Part model, mm, in its own coordinate system. Face numbers are marked on the shaded views. A direction names the side the tool comes from. Round coordinates to 2 decimals unless told otherwise and drop trailing zeros. Order: outer loops, then holes, each group sorted by start corner. A loop starts at its lowest first (then second) coordinate and runs counter-clockwise, first axis right, second up. Notation, with made-up numbers: (-28, -10.5) - (3, -10.5) arc R28 cw to (3, 21.5) - close; hole circle Ø1 at (0, 50.5). An arc over 180 degrees is marked (long way). Answer as a JSON object with one key per item and string values.
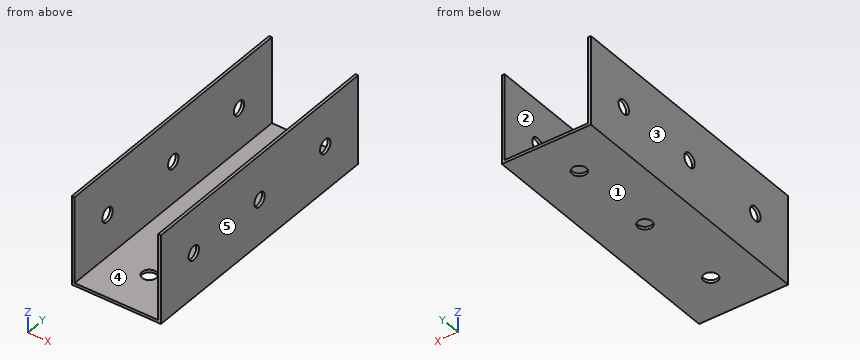
```python
from build123d import *

# Parameters (mm, degrees)
F1_DEPTH = 96
F2_R     = 2.54
F3_DEPTH = 50.8
F4_R     = 2.54
F5_DEPTH = 50.8
F6_R     = 2.54
F7_DEPTH = 25.4


with BuildPart() as f1:
    # F0 (on Front) → F1 (new body)
    with BuildSketch(Plane.XZ):
        Polygon((-15, 15.75), (-16, 15.75), (-16, -16.25), (16, -16.25), (16, 15.75), (15, 15.75), (15, -15.25), (-15, -15.25), align=None)
    extrude(amount=F1_DEPTH)

    # F2 (on face) → F3 (cut)
    with BuildSketch(Plane(origin=(-16, 0, 0), x_dir=(0, -1, 0), z_dir=(-1, 0, 0))):
        with Locations((16, -0.25)):
            Circle(F2_R)
    extrude(amount=-F3_DEPTH, mode=Mode.SUBTRACT)

    # F4 (on face) → F5 (cut)
    with BuildSketch(Plane(origin=(-16, 0, 0), x_dir=(0, -1, 0), z_dir=(-1, 0, 0))):
        with Locations((48, -0.25)):
            Circle(F4_R)
        with Locations((80, -0.25)):
            Circle(F4_R)
    extrude(amount=-F5_DEPTH, mode=Mode.SUBTRACT)

    # F6 (on face) → F7 (cut)
    with BuildSketch(Plane(origin=(0, 0, -16.25), x_dir=(1, 0, 0), z_dir=(0, 0, -1))):
        with Locations((0, 80)):
            Circle(F6_R)
        with Locations((0, 48)):
            Circle(F6_R)
        with Locations((0, 16)):
            Circle(F6_R)
    extrude(amount=-F7_DEPTH, mode=Mode.SUBTRACT)


solid = f1.part
```
Item 1: Cut at C-C (y = -48). Write the cut outline in (x, z), plus the area to 3 significant figures.
Taken from the geometry:
{"outline": "(-16, -16.25) - (-2.54, -16.25) - (-2.54, -15.25) - (-15, -15.25) - (-15, -2.79) - (-16, -2.79) - close; (-16, 2.29) - (-15, 2.29) - (-15, 15.75) - (-16, 15.75) - close; (2.54, -16.25) - (16, -16.25) - (16, -2.79) - (15, -2.79) - (15, -15.25) - (2.54, -15.25) - close; (15, 2.29) - (16, 2.29) - (16, 15.75) - (15, 15.75) - close", "area": "78.8 mm2"}
Item 2: Drop flat-ended pins along their axis: P1, Ø10, axis at y = -46, z = -1, coming from the -X side; P2, Ø6, axis at x = 0, y = -16, coming from the +Z side; P3, Ø3, axis at x = -12, z = 5, coming from the -Y side. Give the stop position or say it passes through.
Taken from the geometry:
{"P1": "x = -16", "P2": "z = -15.25", "P3": "through"}
Item 3: Two-plate mould, pull along X, no slides. Class the marked faces 1, 2 and 3: pulls with the +X half, pulls with the -X half, needs draft (parallel to the pull), parting line crosses it, or undercut.
Taken from the geometry:
{"face 1": "needs draft", "face 2": "undercut", "face 3": "pulls with the -X half"}
Item 4: Probe L1, parallel to Y at x = 0, z = -15.8; L2, parallel to X at y = -16, z = -16; L3, parallel to X at y = -19, z = -13. List the from-to ranges inside material, lowest first. Write a range as from..to.
Taken from the geometry:
{"L1": "-96..-82.54, -77.46..-50.54, -45.46..-18.54, -13.46..0", "L2": "-16..-2.54, 2.54..16", "L3": "-16..-15, 15..16"}
Item 5: Cut at A-A (x = 0). Write the cut outline in (y, z).
Taken from the geometry:
{"outline": "(-96, -16.25) - (-82.54, -16.25) - (-82.54, -15.25) - (-96, -15.25) - close; (-77.46, -16.25) - (-50.54, -16.25) - (-50.54, -15.25) - (-77.46, -15.25) - close; (-45.46, -16.25) - (-18.54, -16.25) - (-18.54, -15.25) - (-45.46, -15.25) - close; (-13.46, -16.25) - (0, -16.25) - (0, -15.25) - (-13.46, -15.25) - close"}
Item 6: Tool access for the marked faces 4 and 5: list every direction of +Z, -Z, +X, -X, +Y, -Y with a clear straight run to the whole face (end or side of a thin tool).
Taken from the geometry:
{"face 4": "+Z, +Y, -Y", "face 5": "+Z, -Z, +X, +Y, -Y"}
Item 7: Cut at B-B (z = 12). Write the cut outline in (x, y), plus the area to 3 significant figures.
Taken from the geometry:
{"outline": "(-16, -96) - (-15, -96) - (-15, 0) - (-16, 0) - close; (15, -96) - (16, -96) - (16, 0) - (15, 0) - close", "area": "192 mm2"}
Item 8: Cut at D-D (y = -87.5). Write the cut outline in (x, z), plus the area to 3 significant figures.
Taken from the geometry:
{"outline": "(-16, -16.25) - (16, -16.25) - (16, 15.75) - (15, 15.75) - (15, -15.25) - (-15, -15.25) - (-15, 15.75) - (-16, 15.75) - close", "area": "94.0 mm2"}
